Can you work these out from the model? Positions are in its coordinate system, mm. A direction names the side the tool comes from. Round coordinates to 2 decimals unless told otherwise and drop trailing zeros. Write each loop counter-clockwise with the first axis right and the second up, starting at its lowest first coordinate (ties: lowest second). Pieces come first, ordered by that corner, then holes. Notation, with made-up numbers: M 30,21 L 87,21 A29 cw 87,56 Z; hole C -1.5,32 d1. An arc over 180 degrees is marked long. Answer in a Markdown table with one row per item. Add a question column.
(1) If we mould it in two halves opening along Y, with no side actions, what happens to faces 5 (the face through (3, -11, 2)), 6 (the face through (3, 0, -10.5)), 7 (the face through (3, 10.5, 0))? For each: released by +Y, released by -Y, zero draft, split by the parting line, or undercut.
(2) For faces 1 (the face through (3, -11, -2)), 2 (the face through (0, -2.5, 7.1)), 3 (the face through (3, 2, 11)), 4 (the face through (3, 11, -2)), which set-ups out of +Z, -Z, +X, -X, +Y, -Y let a thin tool reach every point of the face, with its end or its side?
(3) I'm going to push flat-ended pins straight in: pin 1 (0.6 mm diameter, centred on x = 2.5, z = -11, fed in from +Y); pin 2 (0.6 mm diameter, centred on x = 1.5, y = -11, fed in from -Z); pin 3 (0.9 mm diameter, centred on x = 1.5, y = -11.5, fed in from +Z). Where does each tip first touch, or does it pass through?
(4) If I drill on probe 1 along Z at (x, y) = (2.45, 0); probe 2 along Z at (x, y) = (1.55, 6.25), over which ranges is the centre line in solid material (lowest first)?
(5) Suppose I cut it at A-A, the plane x = 3.1. Write out the boundary of the cut face in (y, z).
(6) Suppose I cut it at B-B, the plane x = 0.75. Write out the boundary of the cut face in (y, z), then the cut area to 3 significant figures.
Autodesk Inventor part; units mm, degrees
ref_plane "Work Plane1" through (35.7071, 0, 0) normal (0, 1, 0) x (-1, 0, 0)
ref_plane "YZ Plane" through (0, 0, 0) normal (1, 0, 0) x (0, 1, 0)
ref_plane "XZ Plane" through (0, 0, 0) normal (0, 1, 0) x (-1, 0, 0)
sketch "Sketch1" plane through (0, 0, 0) normal (0, 0, 1) x (1, 0, 0)
  line L0 (0, 0) -> (5, 0)
  line L1 (0, 0) -> (0, 12.5)
  line L2 (0, 12.5) -> (5, 12.5)
  line L3 (5, 12.5) -> (5, 0)
  line L4 (0, 15) -> (0, -2.5)
  line L5 (-1, 0) -> (6, 0)
  dimension "d1" = 25
  dimension "d2" = 5
revolve "Body" add sketch "Sketch1" angle 360 about axis through (0, 0, 0) along (1, 0, 0)
sketch "Sketch2" plane through (0, 0, 0) normal (-1, 0, 0) x (0, 0, 1)
  circle A0 centre (0, 0) radius 12.5
  point P0 (0, 0)
hole "Thread" at (0, 0, 0) direction (1, 0, 0) diameter 13.917 end through all
chamfer "Chamfer1" distance 2 angle 30 1 edges at (0, -12.5, 0) measured on face at (0, 10.5148, -1.2767)
sketch "Sketch3" plane through (5, 0, 0) normal (1, 0, 0) x (0, 0, -1)
  circle A0 centre (0, 0) radius 12.5
  line L0 (-2, 12.339) -> (-2, 10.5)
  line L1 (-2, 10.5) -> (2, 10.5)
  line L2 (2, 10.5) -> (2, 12.339)
  line L3 (0, -17.5) -> (0, 17.5)
  line L4 (-17.5, 0) -> (17.5, 0)
  dimension "d12" = 2
  dimension "d13" = 2
  dimension "d14" = 10.5
extrude "Groove1" cut sketch "Sketch3" against normal through all contours L2 L1 L3 A0 | L3 L1 L0 A0
pattern_circular "Grooves1" count 4 over 360 about axis through (-10, 0, 0) along (1, 0, 0) of "Groove1"
fillet "Fillet1" radius 0.5 4 edges at (5, 8.8388, 8.8388) (5, 8.8388, -8.8388) (5, -8.8388, -8.8388) (5, -8.8388, 8.8388)
chamfer "Chamfer2" distance 0.375 angle 45 1 edges at (5, 0, -6.9585) measured on face at (5, -8.7255, -5.3872)
chamfer "Chamfer3" distance 0.375 angle 45 1 edges at (0, 0, -6.9585) measured on face at (0, 0.7788, -9.2317)
ref_plane "Work Plane1" through (35.7071, 0, 0) normal (0, 1, 0) x (-1, 0, 0)
equation "\"d1\" = SD2"
equation "\"d2\" = KOH"
equation "\"d12\" = 0.5 * SNB"
equation "\"d13\" = 0.5 * SNB"
equation "\"d14\" = 0.5 * SD2 - SNT"
equation "\"d10\" = -0.5 * LADI + 0.5 * SD2"
equation "\"d11\" = FAWI2"
equation "\"d40\" = -0.5 * LADI + 0.5 * SD2"
equation "\"d18\" = RR"
equation "\"d19\" = 0.025 * NND"
equation "\"d41\" = 0.025 * NND"
equation "\"d21\" = 0.025 * NND"
equation "\"d42\" = 0.025 * NND"
equation "\"NND\" = 15"
equation "\"KOH\" = 5"
equation "\"SD2\" = 25"
equation "\"SNB\" = 4"
equation "\"SNT\" = 2"
equation "\"LADI\" = 21"
equation "\"RR\" = 0.1 * KOH"
equation "\"FAWI2\" = 30deg"
equation "\"THREADDIA\" = 15"
properties part number "KM 02" material "Steel, Mild"
Calculated:
| question | item | result |
|---|---|---|
| 1 | face 5 | zero draft |
| 1 | face 6 | undercut |
| 1 | face 7 | released by +Y |
| 2 | face 1 | +X, -X, -Y |
| 2 | face 2 | +Z, -Z, -X, +Y, -Y |
| 2 | face 3 | +Z, +X, -X |
| 2 | face 4 | +X, -X, +Y |
| 3 | pin 1 | y = 6.46 |
| 3 | pin 2 | z = -6.46 |
| 3 | pin 3 | z = 5.84 |
| 4 | probe 1 | -10.5 to -6.96, 6.96 to 10.5 |
| 4 | probe 2 | -10.83 to -3.06, 3.06 to 10.83 |
| 5 | outline | M -12.34,-2 A12.5 ccw -2,-12.34 L -2,-10.5 L 2,-10.5 L 2,-12.34 A12.5 ccw 12.34,-2 L 10.5,-2 L 10.5,2 L 12.34,2 A12.5 ccw 2,12.34 L 2,10.5 L -2,10.5 L -2,12.34 A12.5 ccw -12.34,2 L -10.5,2 L -10.5,-2 Z; hole C 0,0 d13.92 |
| 6 | outline | M -11.63,-2 A11.8 ccw -2,-11.63 L -2,-10.5 L 2,-10.5 L 2,-11.63 A11.8 ccw 11.63,-2 L 10.5,-2 L 10.5,2 L 11.63,2 A11.8 ccw 2,11.63 L 2,10.5 L -2,10.5 L -2,11.63 A11.8 ccw -11.63,2 L -10.5,2 L -10.5,-2 Z; hole C 0,0 d13.92 |
| 6 | area | 265 mm² |
